Design review of the part built by this model. Coordinates are the model's own, in mm. A direction names the side the tool comes from. Give positions to 0.01 mm unless a question says otherwise; leave off trailing zeros. Order: outer loops, then holes, each group sorted by start corner. A loop starts at its lowest first (then second) coordinate and runs counter-clockwise, first axis right, second up. Notation, with made-up numbers: (-12, 52) -> (18, 52) arc R15 ccw to (18, 59) -> close; hole circle Ø2 at (-3.75, 54.25). An arc over 180 degrees is marked (long way). Return JSON: item names as keys, results as strings.
```python
from build123d import *

# Parameters (mm, degrees)
F1_DEPTH = 63.5
F2_DEPTH = 7.9375
F0_W     = 25.4
F0_H     = 19.05
F3_DEPTH = 25.4
F5_R     = 6.35


with BuildPart() as f1:
    # F0 (on Front) → F1 (new body, symmetric)
    with BuildSketch(Plane.XZ):
        Polygon((-41.275, 9.525), (-41.275, -9.525), (41.275, -9.525), (41.275, 9.525), (22.225, 9.525), align=None)
    extrude(amount=F1_DEPTH, both=True)

    # F0 (on Front) → F2 (join, symmetric)
    with BuildSketch(Plane.XZ):
        with BuildLine():
            add(Edge.make_bspline(
                [(-41.275, 9.525), (-41.1430037548, 34.1428554675), (9.6645992103, 61.636308072), (56.8187902942, 61.9236294583)],
                knots=[0, 0, 0, 0, 111.2440300422, 111.2440300422, 111.2440300422, 111.2440300422], degree=3))
            Line((-41.275, 9.525), (22.225, 9.525))
            Line((22.225, 9.525), (22.225, 27.0002))
            ThreePointArc((22.225, 27.0002), (32.3374716728, 51.5785250653), (56.8187902942, 61.9236294583))
        make_face()
    extrude(amount=F2_DEPTH, both=True)

    # F0 (on Front) → F3 (join, symmetric)
    with BuildSketch(Plane.XZ):
        with BuildLine():
            Line((22.225, 9.525), (41.275, 9.525))
            Line((41.275, 9.525), (41.275, 27.0002))
            ThreePointArc((41.275, 27.0002), (45.9246798487, 38.2255201513), (57.15, 42.8752))
            Line((57.15, 42.8752), (60.325, 42.8752))
            Line((60.325, 42.8752), (60.325, 61.9252))
            Line((60.325, 61.9252), (57.15, 61.9252))
            add(Edge.make_bspline(
                [(56.8187902942, 61.9236294583), (56.9292137967, 61.9243022943), (57.0396172645, 61.9248259369), (57.15, 61.9252)],
                knots=[111.2440300422, 111.2440300422, 111.2440300422, 111.2440300422, 111.5045361635, 111.5045361635, 111.5045361635, 111.5045361635], degree=3))
            ThreePointArc((56.8187902942, 61.9236294583), (32.3374716728, 51.5785250653), (22.225, 27.0002))
            Line((22.225, 27.0002), (22.225, 9.525))
        make_face()
        with Locations((73.025, 52.4002)):
            Rectangle(F0_W, F0_H)
    extrude(amount=F3_DEPTH, both=True)

    # F0 (on Front) → F4 (revolve)
    with BuildSketch(Plane.XZ):
        Polygon((85.725, 66.675), (85.725, 61.9252), (85.802746323, 61.9252), (85.802746323, 42.8752), (85.725, 42.8752), (85.725, 38.1), (111.125, 38.1), (111.125, 66.675), align=None)
    revolve(axis=Axis((85.725, 0, 52.3875), (0, 0, 1)))

    # F5
    f5_edges = [f1.edges().sort_by_distance(p)[0] for p in [
        (-41.275, -63.5, 0),
        (41.275, -63.5, 0),
        (41.275, 63.5, 0),
        (-41.275, 63.5, 0),
    ]]
    fillet(f5_edges, radius=F5_R)


solid = f1.part
```
Item 1: Machinability: for faces 5 (the face through (32.61, 16.55, 51.85)), 6 (the face through (46, 25.4, 42)), 7 (the face through (22.225, -17, 18)), 8 (the face through (86, 0, 38.1)), 9 (the face through (45.8, -0.4, 38.1)), which of the approach directions +Z, -Z, +X, -X, +Y, -Y give a long, thin tool a straight path to every point of the face, cutting with its end or side? Answer none if there is none.
Result set:
{"face 5": "+Z, -X, +Y", "face 6": "+Z, +X, -X, +Y", "face 7": "+Z, -X, -Y", "face 8": "-Z, +X, +Y, -Y", "face 9": "-Z, +Y, -Y"}
Item 2: Add section B-B (x = 89.5). Give the boundary of the cut face in (y, z) (3 decimals), plus the area to 3 significant figures.
Result set:
{"outline": "(-25.118, 38.1) -> (25.118, 38.1) -> (25.118, 66.675) -> (-25.118, 66.675) -> close", "area": "1,440 mm^2"}
Item 3: For pin 1 (14 mm diameter, centred on y = -15.5, z = 18, fed in from -X) (3 decimals); pin 2 (15.5 mm diameter, centred on x = 47.5, z = 28, fed in from +Y); pin 3 (2 mm diameter, centred on x = -12.5, z = 22.5, fed in from +Y), all flat-tipped, find the tip position at first contact; note any pin that passes through.
Result set:
{"pin 1": "stops at x = 22.225", "pin 2": "stops at y = 25.4", "pin 3": "stops at y = 7.94"}
Item 4: Wall thickness on L1, parallel to Y at x = 20, z = 27; L2, parallel to Y at x = 74.5, z = 52; L3, parallel to Z at x = -1, y = -47.5 (3 decimals): over which ranges is each line inside the solid? List them lowest first. Write a range as [from, to].
Result set:
{"L1": "y = [-7.94, 7.94]", "L2": "y = [-25.4, 25.4]", "L3": "z = [-9.525, 9.525]"}
Item 5: Mouldability with a two-part tool opening along X and no side actions: class faces 1 (the face through (41.275, -1, 4)), 2 (the face through (22.225, 17, 18)), 3 (the face through (60, 2, 42.875)), 4 (the face through (0, 63.5, 0)) as released by +X, released by -X, zero draft, split by the parting line, or undercut.
Result set:
{"face 1": "released by +X", "face 2": "released by -X", "face 3": "undercut", "face 4": "zero draft"}
Item 6: Add section A-A (y = -35). Give the boundary of the cut face in (x, z) (3 decimals).
Result set:
{"outline": "(-41.275, -9.525) -> (41.275, -9.525) -> (41.275, 9.525) -> (-41.275, 9.525) -> close"}
